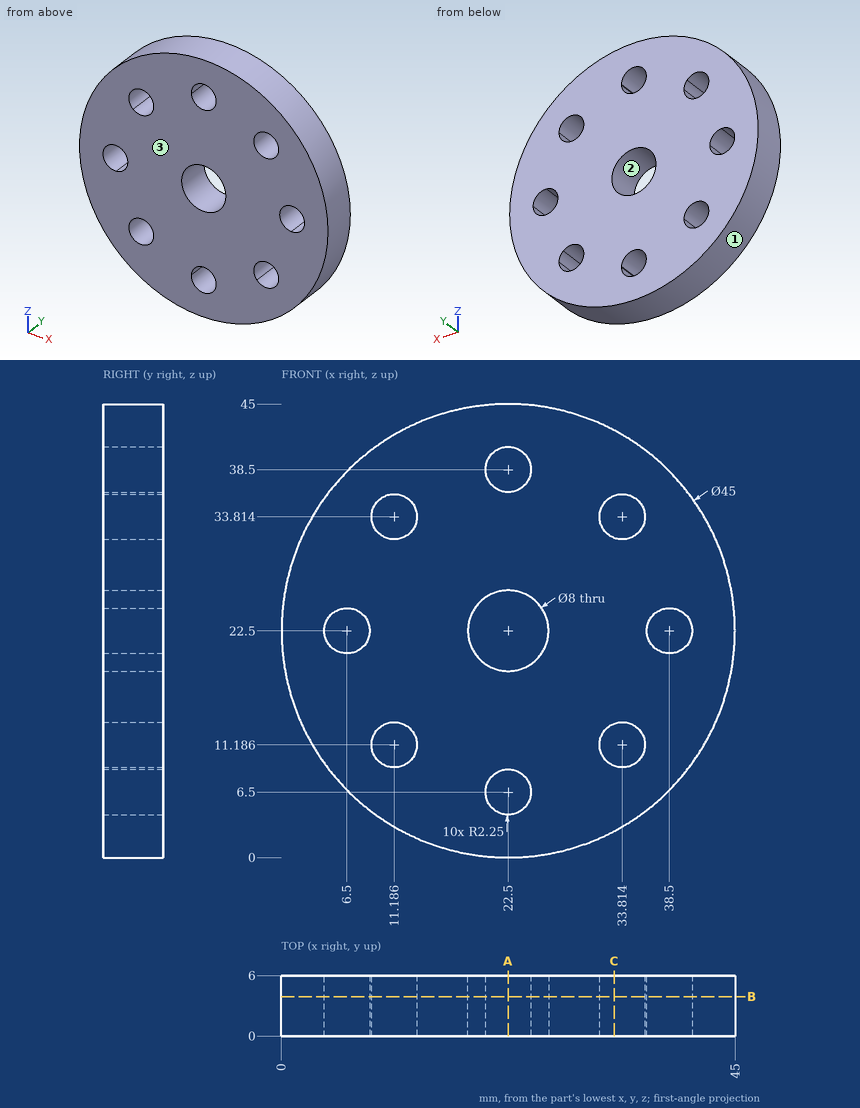
Verification items for this drawing (mm, ordinates from the low corner). Coordinates: 2 decimals unless noted, no trailing zeros. Loops run counter-clockwise (first coordinate to the right, second up) from the corner with the lowest first, then second, coordinate; pieces in that order, holes last. Notation, with made-up numbers: (53.25, 23.25) -> (109.25, 23.25) arc R11 cw to (109.25, 41.25) -> close; hole circle Ø10 at (-14, 62.5). An arc over 180 degrees is marked (long way). Put each result on its own line as item: value.
1. Section check C-C, the plane x = 33. Record the boundary of the cut face in (y, z).
Result set:
outline: (0, 2.6) -> (6, 2.6) -> (6, 9.09) -> (0, 9.09) -> close; (0, 13.28) -> (6, 13.28) -> (6, 31.72) -> (0, 31.72) -> close; (0, 35.91) -> (6, 35.91) -> (6, 42.4) -> (0, 42.4) -> close
2. Section check A-A, the plane x = 22.5. Record the boundary of the cut face in (y, z).
Result set:
outline: (0, 0) -> (6, 0) -> (6, 4.25) -> (0, 4.25) -> close; (0, 8.75) -> (6, 8.75) -> (6, 18.5) -> (0, 18.5) -> close; (0, 26.5) -> (6, 26.5) -> (6, 36.25) -> (0, 36.25) -> close; (0, 40.75) -> (6, 40.75) -> (6, 45) -> (0, 45) -> close
3. Mould release check, pull along Z, two halves, no side actions. Record for the marked faces 1, 2 and 3: pulls with the +Z half, pulls with the -Z half, needs draft (parallel to the pull), parting line crosses it, or undercut.
Result set:
face 1: parting line crosses it
face 2: undercut
face 3: needs draft
4. Gauge pin test, flat ends, axial feed: P1, Ø3, axis at x = 28, y = 4, coming from the +Z side; P2, Ø1.5, axis at y = 3, z = 40, coming from the -X side; P3, Ø1, axis at x = 35, z = 10.5, coming from the -Y side; P4, Ø1.5, axis at y = 4, z = 10.5, coming from the -X side (1 decimal). Record the tip position at first contact, or that the pin passes through.
Result set:
P1: stops at z = 44.64
P2: stops at x = 7.48
P3: passes through
P4: stops at x = 3
5. Section check B-B, the plane y = 3.9. Give the number of separate pieces and of enclosed holes in the cut face, then the cut area to 3 significant figures.
Result set:
separate pieces: 1
enclosed holes: 9
area: 1,410 mm^2
6. Thickness scan on line 1 (Z direction, x = 22.5, y = 4.35); line 2 (X direction, y = 1.5, z = 11.5) (1 decimal); line 3 (Z direction, x = 35, y = 5.15) (1 decimal). Record the ranges inside material, lowest first.
Result set:
line 1: z = 0 to 4.25, 8.75 to 18.5, 26.5 to 36.25, 40.75 to 45
line 2: x = 2.9 to 9, 13.4 to 31.6, 36 to 42.1
line 3: z = 3.8 to 9.3, 13.1 to 31.9, 35.7 to 41.2
